```python
from build123d import *

# Parameters (mm, degrees)
SKIZZE1_R                       = 5
AUFSATZ_LINEAR_AUSTRAGEN1_DEPTH = 20
SKIZZE2_R                       = 2.9
SCHNITT_LINEAR_AUSTRAGEN1_DEPTH = 20
SKIZZE3_R                       = 3
SCHNITT_LINEAR_AUSTRAGEN2_DEPTH = 3
VERRUNDUNG1_R                   = 0.2


with BuildPart() as part:
    # Skizze1 → Aufsatz-Linear austragen1 (new body)
    with BuildSketch(Plane(origin=(0, 0, 0), x_dir=(1, 0, 0), z_dir=(0, 1, 0))):
        with Locations(Location((0, 0, 0), (0, 0, 270))):
            Circle(SKIZZE1_R)
    extrude(amount=AUFSATZ_LINEAR_AUSTRAGEN1_DEPTH)

    # Skizze2 → Schnitt-Linear austragen1 (cut)
    with BuildSketch(Plane(origin=(0, 20, 0), x_dir=(1, 0, 0), z_dir=(0, 1, 0))):
        with Locations(Location((0, 0, 0), (0, 0, 270))):
            Circle(SKIZZE2_R)
    extrude(amount=-SCHNITT_LINEAR_AUSTRAGEN1_DEPTH, mode=Mode.SUBTRACT)

    # Skizze3 → Schnitt-Linear austragen2 (cut)
    with BuildSketch(Plane(origin=(0, 20, 0), x_dir=(1, 0, 0), z_dir=(0, 1, 0))):
        with Locations(Location((0, 0, 0), (0, 0, 270))):
            Circle(SKIZZE3_R)
    extrude(amount=-SCHNITT_LINEAR_AUSTRAGEN2_DEPTH, mode=Mode.SUBTRACT)

    # Verrundung1
    verrundung1_edges = [part.edges().sort_by_distance(p)[0] for p in [
        (0, 20, -5),
    ]]
    fillet(verrundung1_edges, radius=VERRUNDUNG1_R)


solid = part.part
```
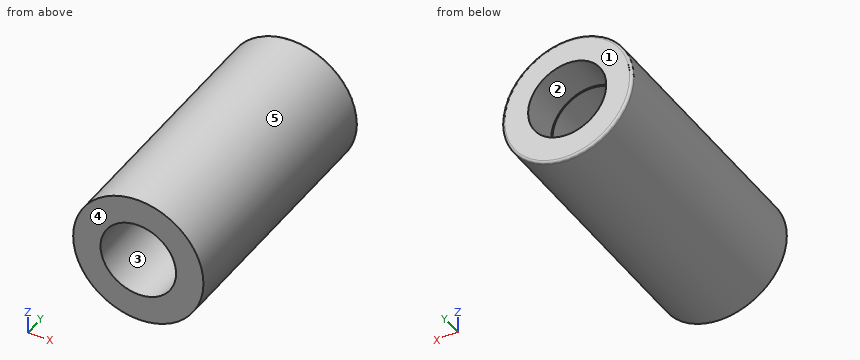
The model under review builds one solid part; all positions refer to its coordinate system, in mm. Face numbers are marked on the shaded views. A direction names the side the tool comes from. Round coordinates to 2 decimals unless told otherwise and drop trailing zeros. Write each loop counter-clockwise with the first axis right and the second up, starting at its lowest first coordinate (ties: lowest second). Pieces come first, ordered by that corner, then holes. Notation, with made-up numbers: (-27, -5.75) - (10, -5.75) arc R22 ccw to (10, 10.25) - close; hole circle Ø3 at (33, 65). An arc over 180 degrees is marked (long way). Answer as CSV lines item,"result". Start each with the question number.
(1) We need section C-C on y = 14.5. State the section outline as (x, z) points, plus the area to 3 significant figures.
(2) We need section A-A on z = 0. State the section outline as (x, y) points.
(3) We need section B-B on y = 18.5. State the section outline as (x, z) points.
(4) To check wall thickness, follow line 1 (X direction, y = 17.8, z = 0); line 2 (X direction, y = 12.5, z = 0); line 3 (Z direction, x = 4, y = 7). State the ranges of each line that lie inside material, in increasing order.
(5) For pin 1 Ø1 at (y, z) = (9, 3) entering from +X, flat-tipped, find the tip position at first contact; note if it passes through.
(6) For the marked faces 1 and 2, list the 3-axis set-ups (+Z, -Z, +X, -X, +Y, -Y) from which the entire face can be reached by the end or side of a thin tool; tool diameter is ignored.
(7) Draft analysis for pull direction X (two halves, no side actions). For the marked faces 3, 4 and 5, state which applies: pulls with the +X half, pulls with the -X half, needs draft (parallel to the pull), parting line crosses it, or undercut.
Worked answers:
1,outline,"circle Ø10 at (0, 0); hole circle Ø5.8 at (0, 0)"
1,area,"52.1 mm²"
2,outline,"(-5, 0) - (-2.9, 0) - (-2.9, 17) - (-3, 17) - (-3, 20) - (-4.8, 20) arc R0.2 ccw to (-5, 19.8) - close; (2.9, 0) - (5, 0) - (5, 19.8) arc R0.2 ccw to (4.8, 20) - (3, 20) - (3, 17) - (2.9, 17) - close"
3,outline,"circle Ø10 at (0, 0); hole circle Ø6 at (0, 0)"
4,line 1,"-5 to -3, 3 to 5"
4,line 2,"-5 to -2.9, 2.9 to 5"
4,line 3,"-3 to 3"
5,pin 1,"x = 4.33"
6,face 1,"+Z, -Z, +X, -X, +Y"
6,face 2,"+Y"
7,face 3,"undercut"
7,face 4,"needs draft"
7,face 5,"parting line crosses it"
